Check sheet for the modelled part. Datum: model origin and axes. Units: mm. Face numbers are marked on the shaded views. A direction names the side the tool comes from. Give positions to 0.01 mm unless a question says otherwise; leave off trailing zeros. Write each loop counter-clockwise with the first axis right and the second up, starting at its lowest first coordinate (ties: lowest second). Pieces come first, ordered by that corner, then holes. Notation, with made-up numbers: (45.25, 50.5) -> (80.25, 50.5) arc R22 ccw to (80.25, 88.5) -> close; hole circle Ø2 at (9, 68.25). An arc over 180 degrees is marked (long way). Answer as a JSON object with one key per item and string values.
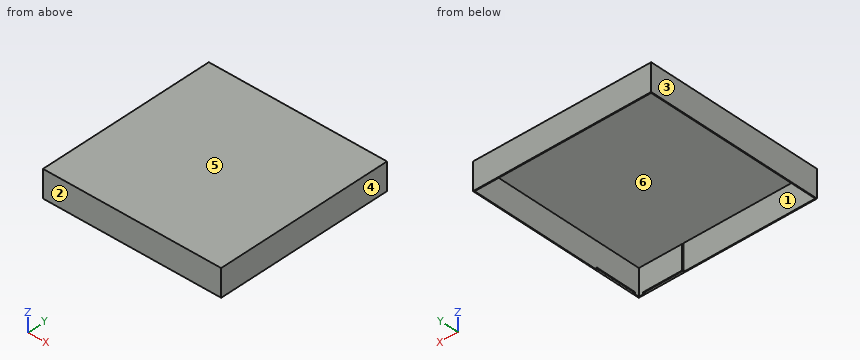
from build123d import *

# Parameters (mm, degrees)
THICKEN1_START       = -150.815
THICKEN1_DEPTH       = 301.63
THICKEN1_2_OUTLINE_W = 298.63
THICKEN1_2_OUTLINE_H = 44.5
THICKEN1_2_DEPTH     = 1.5
THICKEN1_START_2     = 149.315
THICKEN1_3_OUTLINE_W = 298.63
THICKEN1_3_OUTLINE_H = 44.5
THICKEN1_3_DEPTH     = 1.5
CUT_EXTRUDE1_DEPTH   = 3.5
CUT_EXTRUDE2_DEPTH   = 44.5


# Read off the part's stored shape, not the designer's step: Thicken1
with BuildPart() as part:
    # Thicken1 outline → Thicken1 (new body)
    with BuildSketch(Plane(origin=(0, 0, 0), x_dir=(1, 0, 0), z_dir=(0, 1, 0)).offset(THICKEN1_START)):
        Polygon((-150.815, -46), (150.815, -46), (150.815, 0), (149.315, 0), (149.315, -44.5), (-149.315, -44.5), (-149.315, 0), (-150.815, 0), align=None)
    extrude(amount=THICKEN1_DEPTH)

    # Thicken1 2 outline → Thicken1 2 (add)
    with BuildSketch(Plane(origin=(0, 0, 0), x_dir=(1, 0, 0), z_dir=(0, 1, 0)).offset(THICKEN1_START)):
        with Locations((0, -22.25)):
            Rectangle(THICKEN1_2_OUTLINE_W, THICKEN1_2_OUTLINE_H)
    extrude(amount=THICKEN1_2_DEPTH)

    # Thicken1 3 outline → Thicken1 3 (add)
    with BuildSketch(Plane(origin=(0, 0, 0), x_dir=(1, 0, 0), z_dir=(0, 1, 0)).offset(THICKEN1_START_2)):
        with Locations((0, -22.25)):
            Rectangle(THICKEN1_3_OUTLINE_W, THICKEN1_3_OUTLINE_H)
    extrude(amount=THICKEN1_3_DEPTH)

    # Sketch2 → Cut-Extrude1 (cut)
    with BuildSketch(Plane.XY):
        Polygon((147.166053391, -70.458946609), (145.751839828, -71.873160172), (148.8125, -74.933820344), (148.8125, -139.691179656), (139.691179656, -148.8125), (74.933820344, -148.8125), (71.873160172, -145.751839828), (70.458946609, -147.166053391), (74.105393219, -150.8125), (140.519606781, -150.8125), (150.8125, -140.519606781), (150.8125, -74.105393219), align=None)
    extrude(amount=CUT_EXTRUDE1_DEPTH, mode=Mode.SUBTRACT)

    # Sketch3 → Cut-Extrude2 (cut)
    with BuildSketch(Plane.XY):
        with BuildLine():
            Line((73.180697047, -143.737196171), (70.140927125, -146.776966094))
            Line((70.140927125, -146.776966094), (73.115800859, -149.751839828))
            Line((73.115800859, -149.751839828), (75.655768509, -149.751839828))
            ThreePointArc((75.655768509, -149.751839828), (76.458227012, -145.905044907), (73.180697047, -143.737196171))
        make_face()
    extrude(amount=CUT_EXTRUDE2_DEPTH, mode=Mode.SUBTRACT)


solid = part.part
1. Sectioned sample at A-A, the plane z = 36. Enter the section's corners in (x, y) (3 decimals).
Determined:
{"outline": "(-150.815, -150.815) -> (150.815, -150.815) -> (150.815, 150.815) -> (-150.815, 150.815) -> close; hole (-149.315, -149.315) -> (72.679, -149.315) -> (73.116, -149.752) -> (75.656, -149.752) arc R3.5 ccw to (76.038, -149.315) -> (149.315, -149.315) -> (149.315, 149.315) -> (-149.315, 149.315) -> close"}
2. Sectioned sample at B-B, the plane x = -43.5. Enter the section's corners in (y, z) (3 decimals), plus the area to 3 significant figures.
Determined:
{"outline": "(-150.815, 0) -> (-149.315, 0) -> (-149.315, 44.5) -> (149.315, 44.5) -> (149.315, 0) -> (150.815, 0) -> (150.815, 46) -> (-150.815, 46) -> close", "area": "586 mm^2"}
3. Mould release check, pull along X, two halves, no side actions. Record for the marked faces 1, 2, 3 and 4: released by +X, released by -X, zero draft, split by the parting line, or undercut.
Determined:
{"face 1": "undercut", "face 2": "zero draft", "face 3": "released by -X", "face 4": "released by +X"}
4. Go/stop test with flat-tipped pins: P1, Ø1.2, axis at x = 150, y = -124, coming from the -Z side; P2, Ø1.2, axis at x = 116, y = -150.5, coming from the -Z side. Record where each tip stops, or that it passes through.
Determined:
{"P1": "z = 3.5", "P2": "z = 0"}
5. Scan lines: L1, parallel to Y at x = -4.5, z = 30.5 (3 decimals); L2, parallel to Z at x = 108, y = -12.5. Record each from-to range of solid material in increasing order. Write a range as [from, to].
Determined:
{"L1": "[-150.815, -149.315], [149.315, 150.815]", "L2": "[44.5, 46]"}
6. Access from +Z, -Z, +X, -X, +Y, -Y to the whole of each face (thin tool, end or side, straight path). Record for the marked faces 5 and 6.
Determined:
{"face 5": "+Z, +X, -X, +Y, -Y", "face 6": "-Z"}
